```python
from build123d import *

# Parameters (mm, degrees)
SKETCH1_W           = 63.5
SKETCH1_H           = 38.1
SKETCH1_R           = 5.08
SKETCH1_R_2         = 3.2385
SKETCH1_H_2         = 63.5
SKETCH1_R_3         = 1.5
SKETCH1_W_2         = 6.35
SKETCH1_H_3         = 1.5875
BOSS_EXTRUDE1_DEPTH = 3.175
CUT_EXTRUDE1_DEPTH  = 3.175
SKETCH3_R           = 1.5
SKETCH3_W           = 1.5875
SKETCH3_H           = 6.35
CUT_EXTRUDE2_DEPTH  = 3.175
FILLET1_R           = 2.54


with BuildPart() as part:
    # Sketch1 → Boss-Extrude1 (new body)
    # profile 1 of 4: a face of its own
    with BuildSketch(Plane.XY):
        with Locations((31.75, 82.55)):
            Rectangle(SKETCH1_W, SKETCH1_H)
        with Locations((31.75, 88.9)):
            Circle(SKETCH1_R, mode=Mode.SUBTRACT)
    # profile 2 of 4: a face of its own
    with BuildSketch(Plane.XY):
        with Locations((31.75, 82.55)):
            Rectangle(SKETCH1_W, SKETCH1_H)
        with Locations((31.75, 88.9)):
            Circle(SKETCH1_R, mode=Mode.SUBTRACT)
    # profile 3 of 4: a face of its own
    with BuildSketch(Plane.XY):
        with Locations((31.75, 88.9)):
            Circle(SKETCH1_R)
        with Locations((31.75, 88.9)):
            Circle(SKETCH1_R_2, mode=Mode.SUBTRACT)
    # profile 4 of 4: a face of its own
    with BuildSketch(Plane.XY):
        with Locations((31.75, 31.75)):
            Rectangle(SKETCH1_W, SKETCH1_H_2)
        with Locations((31.75, 60.325)):
            Circle(SKETCH1_R_3, mode=Mode.SUBTRACT)
        with Locations((38.1, 60.325)):
            Rectangle(SKETCH1_W_2, SKETCH1_H_3, mode=Mode.SUBTRACT)
        Polygon((27.910940508, 36.891196629), (26.608803371, 35.589059492), (17.62854725, 44.569315613), (18.930684387, 45.87145275), align=None, mode=Mode.SUBTRACT)
        Polygon((45.87145275, 44.569315613), (44.569315613, 45.87145275), (35.589059492, 36.891196629), (36.891196629, 35.589059492), align=None, mode=Mode.SUBTRACT)
        with Locations((25.4, 60.325)):
            Rectangle(SKETCH1_W_2, SKETCH1_H_3, mode=Mode.SUBTRACT)
    extrude(amount=BOSS_EXTRUDE1_DEPTH)

    # Sketch2 → Cut-Extrude1 (cut)
    with BuildSketch(Plane.XY.offset(3.175)):
        Polygon((27.910940508, 36.891196629), (31.75, 33.052137138), (35.589059492, 36.891196629), (44.569315613, 45.87145275), (55.689112862, 56.99125), (7.810887138, 56.99125), (18.930684387, 45.87145275), align=None)
    extrude(amount=-CUT_EXTRUDE1_DEPTH, mode=Mode.SUBTRACT)

    # Sketch3 → Cut-Extrude2 (cut)
    with BuildSketch(Plane.XY.offset(3.175)):
        with Locations((3.81, 12.7)):
            Circle(SKETCH3_R)
        with Locations(Location((59.69, 12.7, 0), (0, 0, 180))):
            Circle(SKETCH3_R)
        with Locations((3.81, 19.05)):
            Rectangle(SKETCH3_W, SKETCH3_H)
        with Locations((3.81, 6.35)):
            Rectangle(SKETCH3_W, SKETCH3_H)
        with Locations((59.69, 6.35)):
            Rectangle(SKETCH3_W, SKETCH3_H)
        with Locations((59.69, 19.05)):
            Rectangle(SKETCH3_W, SKETCH3_H)
    extrude(amount=-CUT_EXTRUDE2_DEPTH, mode=Mode.SUBTRACT)

    # Fillet1
    fillet1_edges = [part.edges().sort_by_distance(p)[0] for p in [
        (0, 101.6, 1.5875),
        (63.5, 101.6, 1.5875),
        (63.5, 0, 1.5875),
        (0, 0, 1.5875),
        (55.689112862, 56.99125, 1.5875),
        (7.810887138, 56.99125, 1.5875),
    ]]
    fillet(fillet1_edges, radius=FILLET1_R)


solid = part.part
```
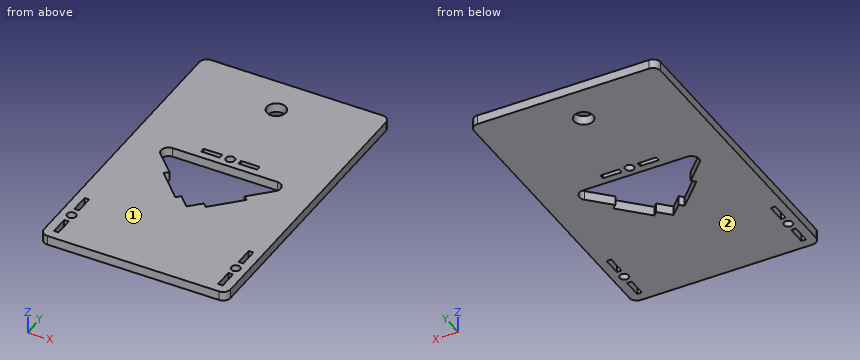
Part model, mm, in its own coordinate system. Face numbers are marked on the shaded views. Give positions to 0.01 mm unless a question says otherwise; leave off trailing zeros. Order: outer loops, then holes, each group sorted by start corner. A loop starts at its lowest first (then second) coordinate and runs counter-clockwise, first axis right, second up. Notation, with made-up numbers: M 7.5,-16 L 27.5,-16 A15 cw 27.5,8 Z; hole C 13.5,55.5 d9. An arc over 180 degrees is marked long. Use a Markdown table: item, result. Add a question column.
(1) Saw through at C-C, the plane y = 39.5. Give the cut face in (x, z) (3 decimals), and give its area (3 significant figures).
(2) Saw through at A-A, the plane y = 12.7. Give the cut face in (x, z) (3 decimals).
(3) Probe line 1 along X through (y, z) = (5, 2.7); line 2 along Y through (x, z) = (59.69, 1.7) (3 decimals); line 3 along Y through (x, z) = (31.75, 2.2) (1 decimal). List the from-to ranges inside material, lowest first. Write a range as [from, to].
(4) Saw through at D-D, the plane z = 1.6. Give the number of separate pieces and of enclosed holes in the cut face, and give its area (3 significant figures).
(5) Mould opens along Z. For the marked faces 1 and 2 say: +Z half, -Z half, draft (parallel to the pull), parting line (faces both ways), or undercut.
(6) Saw through at B-B, the plane x = 25. Give the cut face in (y, z) (3 decimals).
Answer key:
| question | item | result |
|---|---|---|
| 1 | outline | M 0,0 L 22.698,0 L 22.698,3.175 L 0,3.175 Z; M 40.802,0 L 63.5,0 L 63.5,3.175 L 40.802,3.175 Z |
| 1 | area | 144 mm^2 |
| 2 | outline | M 0,0 L 2.31,0 L 2.31,3.175 L 0,3.175 Z; M 5.31,0 L 58.19,0 L 58.19,3.175 L 5.31,3.175 Z; M 61.19,0 L 63.5,0 L 63.5,3.175 L 61.19,3.175 Z |
| 3 | line 1 | [0, 3.02], [4.6, 58.9], [60.48, 63.5] |
| 3 | line 2 | [0, 3.175], [9.525, 11.2], [14.2, 15.875], [22.225, 101.6] |
| 3 | line 3 | [0, 33.1], [57, 58.8], [61.8, 85.7], [92.1, 101.6] |
| 4 | separate pieces | 1 |
| 4 | enclosed holes | 11 |
| 4 | area | 5,730 mm^2 |
| 5 | face 1 | +Z half |
| 5 | face 2 | -Z half |
| 6 | outline | M 0,0 L 37.198,0 L 37.198,3.175 L 0,3.175 Z; M 56.991,0 L 59.531,0 L 59.531,3.175 L 56.991,3.175 Z; M 61.119,0 L 101.6,0 L 101.6,3.175 L 61.119,3.175 Z |
